The listing builds one solid part. Answer for the finished solid, in the listing's coordinates (mm). Give positions to 0.01 mm unless a question says otherwise; leave off trailing zeros. Order: outer loops, then holes, each group sorted by start corner. A loop starts at its lowest first (then second) coordinate and runs counter-clockwise, first axis right, second up. Notation, with made-up numbers: (65.5, 16) -> (69.5, 16) arc R16 cw to (69.5, 37) -> close; hole circle Ø8 at (21, 85). An arc over 180 degrees is marked (long way). Answer as a JSON object with one key per item and string values. Group by question number.
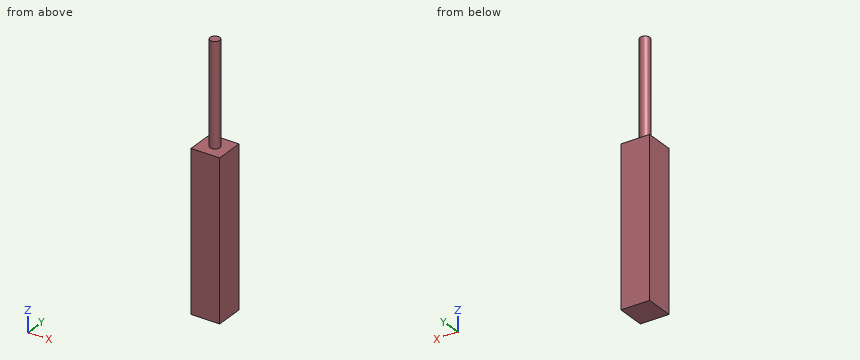
```python
from build123d import *

# Parameters (mm, degrees)
SKETCH_1_W      = 18
SKETCH_1_H      = 18
EXTRUDE_1_DEPTH = 99
SKETCH_2_R      = 3
EXTRUDE_2_DEPTH = 64


with BuildPart() as part:
    # 草图1 → 凸台-拉伸1 (new body)
    with BuildSketch(Plane.XY):
        Rectangle(SKETCH_1_W, SKETCH_1_H)
    extrude(amount=EXTRUDE_1_DEPTH)

    # 草图2 → 凸台-拉伸2 (add)
    with BuildSketch(Plane.XY.offset(99)):
        with Locations(Location((0, 0, 0), (0, 0, 180))):
            Circle(SKETCH_2_R)
    extrude(amount=EXTRUDE_2_DEPTH)


solid = part.part
```
(1) A cutting plane is placed at A-A (y = 0). Determine the outline of the cut face in (x, z), and give its area (3 significant figures).
(2) A cutting plane is placed at C-C (z = 143). Determine the outline of the cut face in (x, y).
(3) Flat-ended cylindrical pins translate along their axes: pin 1 Ø1 at (x, y) = (-5, -6) entering from +Z; pin 2 Ø8 at (x, z) = (-3, 144) entering from +Y. Find the tip coordinate at first contact, or state that the pin passes through.
(4) Find the intervals of material crossed by line 1 along Z through (x, y) = (-6.5, 1.5); line 2 along Y through (x, z) = (2.25, 112); line 3 along X through (y, z) = (2.75, 143), in increasing order. Write a range as [from, to].
(5) A cutting plane is placed at D-D (x = -7). Determine the outline of the cut face in (y, z), and give its area (3 significant figures).
Check sheet entries:
{
 "1": {"outline": "(-9, 0) -> (9, 0) -> (9, 99) -> (3, 99) -> (3, 163) -> (-3, 163) -> (-3, 99) -> (-9, 99) -> close", "area": "2,170 mm2"},
 "2": {"outline": "circle Ø6 at (0, 0)"},
 "3": {"pin 1": "stops at z = 99", "pin 2": "stops at y = 3"},
 "4": {"line 1": "z = [0, 99]", "line 2": "y = [-1.98, 1.98]", "line 3": "x = [-1.2, 1.2]"},
 "5": {"outline": "(-9, 0) -> (9, 0) -> (9, 99) -> (-9, 99) -> close", "area": "1,780 mm2"}
}
